Design review of the part shown in the three views and the two pictorial views. Dimensions are in mm from the part's minimum x, y and z. A direction names the side the tool comes from. Round coordinates to 2 decimals unless told otherwise and drop trailing zeros. Write each loop counter-clockwise with the first axis right and the second up, starting at its lowest first coordinate (ties: lowest second). Pieces come first, ordered by that corner, then holes. Notation, with made-up numbers: (-10, 34.25) - (33, 34.25) arc R16 cw to (33, 39.25) - close; hole circle Ø9 at (-32.75, 0.5). An arc over 180 degrees is marked (long way). Use one line per item in the form item = value.
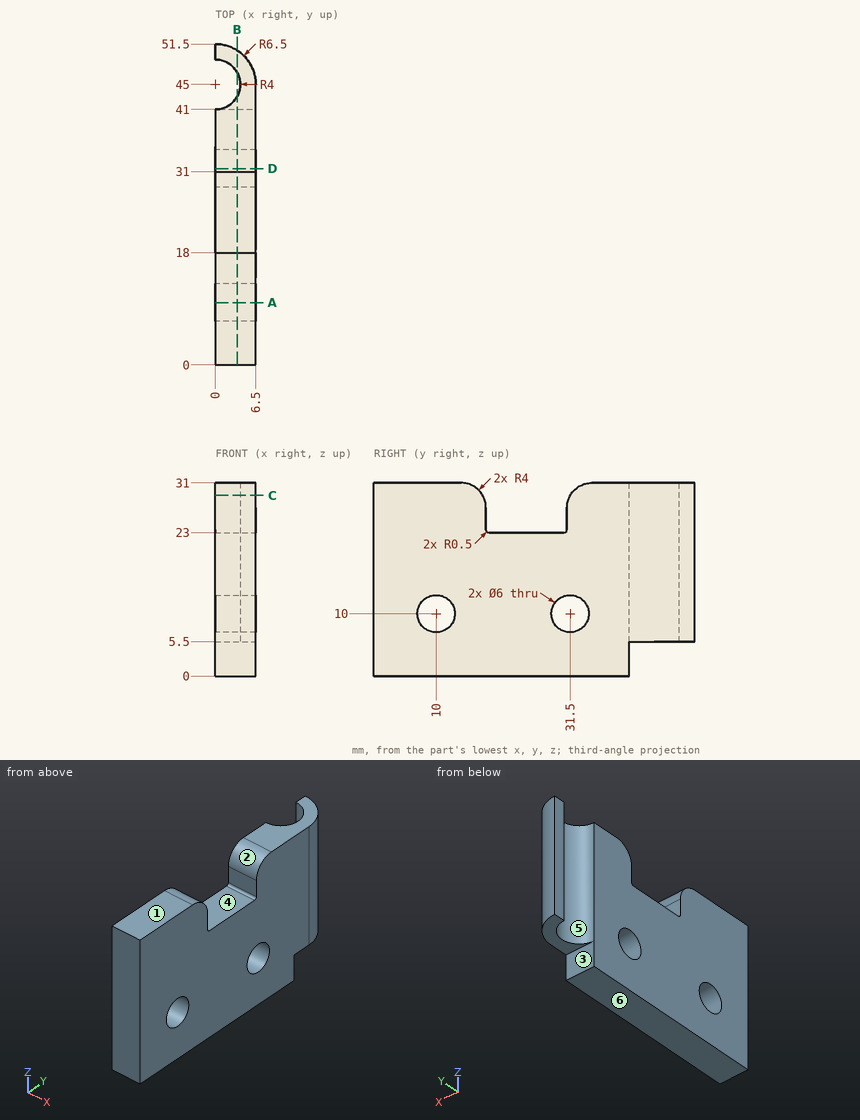
Q1. We need section D-D on y = 31.5. Write out the cut boundary in (x, z), then the cut area to 3 significant figures.
Calculated:
outline = (0, 0) - (6.5, 0) - (6.5, 7) - (0, 7) - close; (0, 13) - (6.5, 13) - (6.5, 28.94) - (0, 28.94) - close
area = 149 mm2
Q2. We need section A-A on y = 10. Write out the cut boundary in (x, z), then the cut area to 4 significant figures.
Calculated:
outline = (0, 0) - (6.5, 0) - (6.5, 7) - (0, 7) - close; (0, 13) - (6.5, 13) - (6.5, 31) - (0, 31) - close
area = 162.5 mm2
Q3. For P1, Ø1, axis at x = 2, z = 24.5, coming from the +Y side; P2, Ø2, axis at y = 42.5, z = 5, coming from the +X side; P3, Ø3.5, axis at x = 4.5, y = 47, coming from the -Z side; P4, Ø1.6, axis at x = 2.5, z = 3.5, coming from the +Y side, all flat-tipped, find the tip position at first contact; note any pin that passes through.
Calculated:
P1 = 51.32
P2 = 6.5
P3 = 5.5
P4 = 41
Q4. Draft analysis for pull direction Y (two halves, no side actions). For the marked faces 3, 4, 5 and 6, state which applies: released by +Y, released by -Y, zero draft, split by the parting line, or undercut.
Calculated:
face_3 = released by +Y
face_4 = undercut
face_5 = undercut
face_6 = zero draft
Q5. Machinability: for the marked faces 1 and 2, which of the approach directions +Z, -Z, +X, -X, +Y, -Y give a long, thin tool a straight path to every point of the face, cutting with its end or side? Answer none if there is none.
Calculated:
face_1 = +Z, +X, -X, +Y, -Y
face_2 = +Z, +X, -X
Q6. We need section C-C on z = 29. Write out the cut boundary in (x, y).
Calculated:
outline = (0, 0) - (6.5, 0) - (6.5, 17.46) - (0, 17.46) - close; (0, 31.54) - (6.5, 31.54) - (6.5, 45) arc R6.5 ccw to (0, 51.5) - (0, 49) arc R4 cw to (0, 41) - close
Q7. We need section B-B on x = 3.5. Write out the cut boundary in (y, z), then the cut area to 3 significant figures.
Calculated:
outline = (0, 0) - (41, 0) - (41, 5.5) - (43.06, 5.5) - (43.06, 31) - (35, 31) arc R4 ccw to (31, 27) - (31, 23.5) arc R0.5 cw to (30.5, 23) - (18.5, 23) arc R0.5 cw to (18, 23.5) - (18, 27) arc R4 ccw to (14, 31) - (0, 31) - close; (46.94, 5.5) - (50.48, 5.5) - (50.48, 31) - (46.94, 31) - close; hole circle Ø6 at (10, 10); hole circle Ø6 at (31.5, 10)
area = 1,250 mm2
Q8. To check wall thickness, follow line 1 along Y through (x, z) = (1.5, 10); line 2 along Y through (x, z) = (3.25, 10); line 3 along Y through (x, z) = (4.5, 10). State the ranges of each line that lie inside material, in increasing order. Write a range as from..to.
Calculated:
line_1 = 0..7, 13..28.5, 34.5..41.29, 48.71..51.32
line_2 = 0..7, 13..28.5, 34.5..42.67, 47.33..50.63
line_3 = 0..7, 13..28.5, 34.5..49.69
